from build123d import *

# Parameters (mm, degrees)
SZKIC1_R                    = 14.5
SZKIC1_R_2                  = 5
DODANIE_WYCI_GNI_CIE1_DEPTH = 15
M6_TAPPED_HOLE1_D           = 5
DODANIE_WYCI_GNI_CIE3_START = -25
DODANIE_WYCI_GNI_CIE3_DEPTH = 25
WYTNIJ_WYCI_GNI_CIE2_DEPTH  = 10
WYTNIJ_WYCI_GNI_CIE4_DEPTH  = 20
SFAZOWANIE4_SIZE            = 10
WYTNIJ_WYCI_GNI_CIE5_DEPTH  = 5
SZKIC17_5_R                 = 7.5
WYTNIJ_WYCI_GNI_CIE6_DEPTH  = 163.311542951


with BuildPart() as part:
    # Szkic1 → Dodanie-wyci_gni_cie1 (new, symmetric)
    with BuildSketch(Plane(origin=(0, 0, 0), x_dir=(0, 0, -1), z_dir=(1, 0, 0))):
        with BuildLine():
            Line((62.076569761, 109.385977671), (65.40069858, 86.060032436))
            ThreePointArc((65.40069858, 86.060032436), (67.080888035, 80.867469231), (70.408575711, 76.541704099))
            ThreePointArc((70.408575711, 76.541704099), (81.115709466, 65.086416999), (89.978943384, 52.151603499))
            ThreePointArc((89.978943384, 52.151603499), (92.32041193, 40.919666146), (87.495806927, 30.50995538))
            ThreePointArc((87.495806927, 30.50995538), (75.419960244, 0), (87.495806927, -30.50995538))
            ThreePointArc((87.495806927, -30.50995538), (92.32041193, -40.919666146), (89.978943384, -52.151603499))
            ThreePointArc((89.978943384, -52.151603499), (77.589025222, -69.25274843), (62, -83.498502981))
            Line((62, -83.498502981), (62, -100))
            ThreePointArc((62, -100), (58.828108774, -114.988630917), (49.856267202, -127.407407407))
            ThreePointArc((49.856267202, -127.407407407), (46.738768646, -129.329364235), (43.138357147, -130))
            Line((43.138357147, -130), (25, -130))
            Line((25, -130), (-25, -130))
            Line((-25, -130), (-43.138357147, -130))
            ThreePointArc((-43.138357147, -130), (-46.738768646, -129.329364235), (-49.856267202, -127.407407407))
            ThreePointArc((-49.856267202, -127.407407407), (-58.828108774, -114.988630917), (-62, -100))
            Line((-62, -100), (-62, -83.498502981))
            ThreePointArc((-62, -83.498502981), (-77.589025222, -69.25274843), (-89.978943384, -52.151603499))
            ThreePointArc((-89.978943384, -52.151603499), (-92.32041193, -40.919666146), (-87.495806927, -30.50995538))
            ThreePointArc((-87.495806927, -30.50995538), (-75.419960244, 0), (-87.495806927, 30.50995538))
            ThreePointArc((-87.495806927, 30.50995538), (-92.32041193, 40.919666146), (-89.978943384, 52.151603499))
            ThreePointArc((-89.978943384, 52.151603499), (-81.115709466, 65.086416999), (-70.408575711, 76.541704099))
            ThreePointArc((-70.408575711, 76.541704099), (-67.080888035, 80.867469231), (-65.40069858, 86.060032436))
            Line((-65.40069858, 86.060032436), (-62.076569761, 109.385977671))
            ThreePointArc((-62.076569761, 109.385977671), (-54.044566654, 124.12820267), (-38.316621209, 130))
            Line((-38.316621209, 130), (38.316621209, 130))
            ThreePointArc((38.316621209, 130), (54.044566654, 124.12820267), (62.076569761, 109.385977671))
        make_face()
        Circle(SZKIC1_R, mode=Mode.SUBTRACT)
        with Locations(Location((74.189369185, -43, 0), (0, 0, 180))):
            Circle(SZKIC1_R_2, mode=Mode.SUBTRACT)
        with Locations(Location((74.189369185, 43, 0), (0, 0, 180))):
            Circle(SZKIC1_R_2, mode=Mode.SUBTRACT)
        with BuildLine():
            Line((-25, -84), (25, -84))
            ThreePointArc((25, -84), (41, -100), (25, -116))
            Line((25, -116), (-25, -116))
            ThreePointArc((-25, -116), (-41, -100), (-25, -84))
        make_face(mode=Mode.SUBTRACT)
    extrude(amount=DODANIE_WYCI_GNI_CIE1_DEPTH, both=True)

    # M6 Tapped Hole1 (through all)
    with Locations(Plane(origin=(15, 0, 0), x_dir=(0, 0, -1), z_dir=(1, 0, 0))):
        with Locations((-29.489576473, 100), (50.510423527, 100)):
            Hole(M6_TAPPED_HOLE1_D / 2)

    # Szkic5 → Dodanie-wyci_gni_cie3 (add)
    with BuildSketch(Plane.ZY.offset(-15).offset(DODANIE_WYCI_GNI_CIE3_START)):
        with BuildLine():
            Line((-40.419960244, -6), (-44.419960244, -10))
            Line((-44.419960244, -10), (-76.556013712, -10))
            ThreePointArc((-76.556013712, -10), (-75.704884126, -5.032161998), (-75.419960244, 0))
            Line((-75.419960244, 0), (-44.419960244, 0))
            Line((-44.419960244, 0), (-40.419960244, -4))
            Line((-40.419960244, -4), (-40.419960244, -6))
        make_face()
    extrude(amount=DODANIE_WYCI_GNI_CIE3_DEPTH)

    # Szkic12 → Wytnij-wyci_gni_cie2 (cut)
    with BuildSketch(Plane(origin=(15, 0, 0), x_dir=(0, 0, -1), z_dir=(1, 0, 0))):
        with BuildLine():
            Line((30.510423527, 105), (-9.489576473, 105))
            ThreePointArc((-9.489576473, 105), (-14.489576473, 100), (-9.489576473, 95))
            Line((-9.489576473, 95), (30.510423527, 95))
            ThreePointArc((30.510423527, 95), (35.510423527, 100), (30.510423527, 105))
        make_face()
    extrude(amount=-WYTNIJ_WYCI_GNI_CIE2_DEPTH, mode=Mode.SUBTRACT)

    # Szkic16 → Wytnij-wyci_gni_cie4 (cut)
    with BuildSketch(Plane(origin=(15, 0, 0), x_dir=(0, 0, -1), z_dir=(1, 0, 0))):
        with BuildLine():
            Line((-43.138357147, -130), (43.138357147, -130))
            ThreePointArc((43.138357147, -130), (46.738768646, -129.329364235), (49.856267202, -127.407407407))
            ThreePointArc((49.856267202, -127.407407407), (58.828108774, -114.988630917), (62, -100))
            Line((62, -100), (62, -83.498502981))
            ThreePointArc((62, -83.498502981), (69.784912958, -77.110738056), (76.915538092, -70))
            Line((76.915538092, -70), (-76.915538092, -70))
            ThreePointArc((-76.915538092, -70), (-69.784912958, -77.110738056), (-62, -83.498502981))
            Line((-62, -83.498502981), (-62, -100))
            ThreePointArc((-62, -100), (-58.828108774, -114.988630917), (-49.856267202, -127.407407407))
            ThreePointArc((-49.856267202, -127.407407407), (-46.738768646, -129.329364235), (-43.138357147, -130))
        make_face()
        with BuildLine():
            Line((-25, -116), (25, -116))
            ThreePointArc((25, -116), (41, -100), (25, -84))
            Line((25, -84), (-25, -84))
            ThreePointArc((-25, -84), (-41, -100), (-25, -116))
        make_face(mode=Mode.SUBTRACT)
    extrude(amount=-WYTNIJ_WYCI_GNI_CIE4_DEPTH, mode=Mode.SUBTRACT)

    # Sfazowanie4
    sfazowanie4_edges = [part.edges().sort_by_distance(p)[0] for p in [
        (15, -70, 0),
    ]]
    chamfer(sfazowanie4_edges, length=SFAZOWANIE4_SIZE)

    # Szkic17 → Wytnij-wyci_gni_cie5 (cut)
    with BuildSketch(Plane(origin=(15, 0, 0), x_dir=(0, 0, -1), z_dir=(1, 0, 0))):
        with BuildLine():
            Line((-31.578571429, -10.936663672), (-45.292857143, -8.957177035))
            ThreePointArc((-45.292857143, -8.957177035), (-53.050000001, 0), (-45.292857143, 8.957177034))
            Line((-45.292857143, 8.957177034), (-31.578571428, 10.93666367))
            ThreePointArc((-31.578571428, 10.93666367), (-22.462605729, 8.080234378), (-18.98012619, -0.815402484))
            ThreePointArc((-18.98012619, -0.815402484), (-23.079412621, -8.614404817), (-31.578571429, -10.936663672))
        make_face()
    extrude(amount=-WYTNIJ_WYCI_GNI_CIE5_DEPTH, mode=Mode.SUBTRACT)

    # Szkic17_5 → Wytnij-wyci_gni_cie6 (cut, through all)
    with BuildSketch(Plane(origin=(15, 0, 0), x_dir=(0, 0, -1), z_dir=(1, 0, 0))):
        with Locations(Location((-30, -1e-09, 0), (0, 0, 180))):
            Circle(SZKIC17_5_R)
    extrude(amount=-WYTNIJ_WYCI_GNI_CIE6_DEPTH, mode=Mode.SUBTRACT)


solid = part.part
Work out the finished part from the listing and answer in its coordinate system (mm). A direction names the side the tool comes from. Give positions to 0.01 mm unless a question says otherwise; leave off trailing zeros. Loops run counter-clockwise (first coordinate to the right, second up) from the corner with the lowest first, then second, coordinate; pieces in that order, holes last. Notation, with made-up numbers: M 43,80 L 79,80 A15 cw 79,101 Z; hole C -20.75,-33 d4. An arc over 180 degrees is marked long. Use CSV: the item, a comma, the result in double quotes.
1) Find section D-D on x = 27. Write down the section's boundary in (y, z).
Answer:
outline,"M -10,-76.56 A44.58 cw 0,-75.42 L 0,-44.42 L -4,-40.42 L -6,-40.42 L -10,-44.42 Z"
2) Find section A-A on y = -43. Write down the section's boundary in (x, z), plus the area to 3 significant figures.
Answer:
outline,"M -15,-92.44 L 15,-92.44 L 15,-79.19 L -15,-79.19 Z; M -15,-69.19 L 15,-69.19 L 15,92.44 L -15,92.44 Z"
area,"5,250 mm^2"
3) Consider L1, parallel to Y at x = -0.5, z = 30; L2, parallel to Y at x = -7, z = 0; L3, parallel to Y at x = -1, z = 0. Determine where each line is inside the solid, lowest interval first.
Answer:
L1,"-70 to -7.5, 7.5 to 97.55, 102.45 to 130"
L2,"-130 to -116, -84 to -14.5, 14.5 to 130"
L3,"-70 to -14.5, 14.5 to 130"
4) Determine the mould class of faces 6 (the cylindrical face through (0.21, 65.258, -80.978)), 7 (the flat face through (-10, -130, -1)), 8 (the cylindrical face through (10.07, 99.89, -35.51)) for opening direction Z: released by +Z, released by -Z, zero draft, split by the parting line, or undercut.
Answer:
face 6,"released by -Z"
face 7,"zero draft"
face 8,"undercut"
5) Find section C-C on z = 0. Write down the section's boundary in (x, y).
Answer:
outline,"M -15,-130 L -5,-130 L -5,-116 L -15,-116 Z; M -15,-84 L -5,-84 L -5,-70 L 5,-70 L 15,-60 L 15,-14.5 L -15,-14.5 Z; M -15,14.5 L 15,14.5 L 15,95 L 5,95 L 5,105 L 15,105 L 15,130 L -15,130 Z"
6) Given P1, Ø8, axis at x = 8, z = -20, coming from the -Y side; P2, Ø12, axis at y = 54.5, z = -27, coming from the +X side; P3, Ø11, axis at x = -8, y = -90, coming from the +Z side, each flat-ended and moving along its own axis, determine where each tip first touches the part or whether it passes through.
Answer:
P1,"y = -70"
P2,"x = 15"
P3,"z = 62"
7) Which of the six approach directions +Z, -Z, +X, -X, +Y, -Y give full straight-line access (tool end or side, diameter ignored) to faces 1 (the flat face through (12.535, 9.933, 38.532)), 2 (the cylindrical face through (-9.93, -115.19, 58.74)), 3 (the flat face through (0, -70, -1)), 4 (the flat face through (-10, -84, 0)), 5 (the flat face through (0.21, 97.56, 63.76))?
Answer:
face 1,"+X"
face 2,"+Z, +X, -X, -Y"
face 3,"+Z, -Z, +X, -Y"
face 4,"+X, -X"
face 5,"+Z, +X, -X, +Y"
8) Find section B-B on x = -2. Write down the section's boundary in (y, z), plus the area to 3 significant figures.
Answer:
outline,"M -70,-76.92 A104 ccw -52.15,-89.98 A18.25 ccw -30.51,-87.5 A44.58 cw 30.51,-87.5 A18.25 ccw 52.15,-89.98 A104 ccw 76.54,-70.41 A16 cw 86.06,-65.4 L 109.39,-62.08 A24 ccw 130,-38.32 L 130,38.32 A24 ccw 109.39,62.08 L 86.06,65.4 A16 cw 76.54,70.41 A104 ccw 52.15,89.98 A18.25 ccw 30.51,87.5 A44.58 cw -30.51,87.5 A18.25 ccw -52.15,89.98 A104 ccw -70,76.92 Z; hole C -43,-74.19 d10; hole C 0,0 d29; hole C 0,30 d15; hole C 43,-74.19 d10; hole C 100,-50.51 d5; hole C 100,29.49 d5"
area,"30,100 mm^2"
